from build123d import *

# Parameters (mm, degrees)
F1_DEPTH  = 127
F3_DEPTH  = 19.05
F5_DEPTH  = 19.05
F6_R      = 3.0369743136
F7_DEPTH  = 25.4
F8_W      = 4.4003706425
F8_H      = 12.9362940788
F8_W_2    = 4.6123838983
F8_H_2    = 11.268997401
F9_DEPTH  = 7.62
F8_W_3    = 58.9885585941
F8_H_3    = 15.6373567879
F10_DEPTH = 12.7
F12_DEPTH = 25.4


with BuildPart() as f1:
    # F0 (on Top) → F1 (new body)
    with BuildSketch(Plane.XY):
        Polygon((-19.05, 3.81), (-19.05, 19.05), (19.05, 19.05), (19.05, -19.05), (3.81, -19.05), (0.0297182501, -19.05), (3.81, -22.86), (22.86, -22.86), (22.86, 22.86), (-22.6519722492, 22.86), (-22.6519722492, 3.81), (-19.05, 0.1797112604), align=None)
        Polygon((3.81, -19.05), (-19.05, 3.81), (-19.05, 0.1797112604), (0.0297182501, -19.05), align=None)
    extrude(amount=F1_DEPTH)

    # F2 (on face) → F3 (join)
    with BuildSketch(Plane.YZ.offset(22.86)):
        Polygon((-22.86, 0), (-22.86, 78.74), (-101.6, 0), align=None)
    extrude(amount=-F3_DEPTH)

    # F4 (on face) → F5 (join)
    with BuildSketch(Plane(origin=(0, 22.86, 0), x_dir=(-1, 0, 0), z_dir=(0, 1, 0))):
        Polygon((101.6, 0), (22.6519722492, 78.9480277508), (22.6519722492, 0), align=None)
    extrude(amount=-F5_DEPTH)

    # F6 (on face) → F7 (cut)
    with BuildSketch(Plane(origin=(-9.5097324965, -9.4355559587, 0), x_dir=(0.7043328456, -0.7098698772, 0), z_dir=(-0.7098698772, -0.7043328456, 0))):
        with Locations((0, 63.7570247054)):
            Circle(F6_R)
    extrude(amount=-F7_DEPTH, mode=Mode.SUBTRACT)

    # F8 (on face) → F9 (join)
    with BuildSketch(Plane(origin=(0, 22.86, 0), x_dir=(-1, 0, 0), z_dir=(0, 1, 0))):
        with Locations((-16.0567304119, 94.7479456663)):
            Rectangle(F8_W, F8_H)
        with Locations((-7.4986156542, 94.7479456663)):
            Rectangle(F8_W_2, F8_H)
        with Locations((-16.0567304119, 57.8655012995)):
            Rectangle(F8_W, F8_H_2)
        with Locations((-7.4986156542, 57.8655012995)):
            Rectangle(F8_W_2, F8_H_2)
    extrude(amount=F9_DEPTH)

    # F8 (on face) → F10 (join)
    with BuildSketch(Plane(origin=(0, 22.86, 0), x_dir=(-1, 0, 0), z_dir=(0, 1, 0))):
        with Locations((30.81879206, 30.5291432887)):
            Rectangle(F8_W_3, F8_H_3)
    extrude(amount=F10_DEPTH)

    # F11 (on face) → F12 (cut)
    with BuildSketch(Plane.XY.offset(38.3478216827)):
        with BuildLine():
            ThreePointArc((-49.531262368, 35.56), (-45.6181932241, 27.0444772391), (-41.7051240802, 35.56))
            Line((-41.7051240802, 35.56), (-49.531262368, 35.56))
        make_face()
        with BuildLine():
            ThreePointArc((-30.81879206, 35.56), (-26.5684658661, 27.6497786466), (-22.3181396723, 35.56))
            Line((-22.3181396723, 35.56), (-30.81879206, 35.56))
        make_face()
        with BuildLine():
            Line((-4.8403558321, 35.56), (-10.8519690111, 35.56))
            ThreePointArc((-10.8519690111, 35.56), (-7.8461624216, 27.8403776177), (-4.8403558321, 35.56))
        make_face()
    extrude(amount=-F12_DEPTH, mode=Mode.SUBTRACT)


solid = f1.part
CAD build for the part. Positions are in the model's coordinates, mm. A direction names the side the tool comes from. Round coordinates to 2 decimals unless told otherwise and drop trailing zeros. Loops run counter-clockwise (first coordinate to the right, second up) from the corner with the lowest first, then second, coordinate; pieces in that order, holes last. Notation, with made-up numbers: M 80.25,-37.5 L 108.25,-37.5 A24 cw 108.25,-11.5 Z; hole C 2.5,82.5 d9. An arc over 180 degrees is marked long. One line per question, with ' | ' between items. Start each with the question number.
Item 1: Wall check: line 1 (Y direction, x = 17, z = 88); line 2 (X direction, y = -34.5, z = 53). Give the ranges that are in metal, low to high.
Item 2: Which spindle directions (+Z, -Z, +X, -X, +Y, -Y) get a long thin tool onto all of the face, cutting with end or side? Do faces 5 (the flat face through (9.805, 27, 58)), 6 (the flat face through (-30, 28, 38.348)), 7 (the flat face through (5.192, 27, 58)), 8 (the flat face through (16, 27, 88.28)), 9 (the flat face through (13, -22.86, 103)). Say none if no direction does.
Item 3: Cut at B-B, the plane y = -15. Write the cut outline in (x, z), plus the area to 3 significant figures.
Item 4: Cut at D-D, the plane z = 41.5. Write the cut outline in (x, y).
Item 5: Two-plate mould, pull along Y, no slides. Class faces 1 (the cylindrical face through (-7.995, 27.843, 30.639)), 2 (the flat face through (-10, -5.24, 62.61)), 3 (the flat face through (13.5, -61.7, 39.9)), 4 (the flat face through (-30, 28, 22.71)): pulls with the +Y half, pulls with the -Y half, needs draft (parallel to the pull), parting line crosses it, or undercut.
Item 6: Cut at A-A, the plane z = 13.5. Write the cut outline in (x, y), plus the area to 3 significant figures.
Item 7: Cut at C-C, the plane x = -38. Write the cut outline in (y, z), plus the area to 3 significant figures.
Item 8: Pin check, flat tips, straight feed: pin 1 Ø23.5 at (y, z) = (-48.5, 33.5) entering from -X; pin 2 Ø6 at (y, z) = (26, 57.5) entering from -X; pin 3 Ø1.3 at (x, y) = (15, 28) entering from -Z; pin 4 Ø1.5 at (x, y) = (-70, 2.5) entering from -Z. Stop position of each tip, or through.
Responses:
1) line 1: y = -22.86 to -19.05, 19.05 to 22.86 | line 2: x = 3.81 to 22.86
2) face 5: +Z, -Z, +Y | face 6: +Z, +X, -X, +Y | face 7: +Z, -Z, -X, +Y | face 8: +X, -X, +Y | face 9: +Z, +X, -X, -Y
3) outline: M -3.99,0 L -0.24,0 L -0.24,127 L -3.99,127 Z; M 19.05,0 L 22.86,0 L 22.86,127 L 19.05,127 Z | area: 960 mm²
4) outline: M -60.1,3.81 L -22.65,3.81 L 3.81,-22.86 L 3.81,-60.1 L 22.86,-60.1 L 22.86,22.86 L -60.1,22.86 Z; hole M -19.05,3.81 L 3.81,-19.05 L 19.05,-19.05 L 19.05,19.05 L -19.05,19.05 Z
5) face 1: undercut | face 2: undercut | face 3: pulls with the -Y half | face 4: needs draft
6) outline: M -88.1,3.81 L -22.65,3.81 L 3.81,-22.86 L 3.81,-88.1 L 22.86,-88.1 L 22.86,22.86 L -88.1,22.86 Z; hole M -19.05,3.81 L 3.81,-19.05 L 19.05,-19.05 L 19.05,19.05 L -19.05,19.05 Z | area: 3,030 mm²
7) outline: M 3.81,0 L 22.86,0 L 22.86,22.71 L 35.56,22.71 L 35.56,38.35 L 22.86,38.35 L 22.86,63.6 L 3.81,63.6 Z | area: 1,410 mm²
8) pin 1: stops at x = 3.81 | pin 2: stops at x = 5.19 | pin 3: stops at z = 52.23 | pin 4: passes through
